from build123d import *

# Parameters (mm, degrees)
SKETCH1_W           = 114.3
SKETCH1_H           = 9.525
BOSS_EXTRUDE1_DEPTH = 3.175
SKETCH2_W           = 9.525
SKETCH2_H           = 63.5
BOSS_EXTRUDE2_DEPTH = 3.175
SKETCH3_W           = 9.525
SKETCH3_H           = 3.81
BOSS_EXTRUDE3_DEPTH = 12.7
SKETCH4_W           = 114.3
SKETCH4_H           = 3.81
BOSS_EXTRUDE4_DEPTH = 3.175
CHAMFER1_SIZE       = 12.7
CHAMFER2_SIZE       = 6.35


with BuildPart() as part:
    # Sketch1 → Boss-Extrude1 (new body)
    with BuildSketch(Plane(origin=(0, 0, 0), x_dir=(1, 0, 0), z_dir=(0, 1, 0))):
        Rectangle(SKETCH1_W, SKETCH1_H)
    extrude(amount=BOSS_EXTRUDE1_DEPTH)

    # Sketch2 → Boss-Extrude2 (add)
    with BuildSketch(Plane(origin=(0, 3.175, 0), x_dir=(1, 0, 0), z_dir=(0, 1, 0))):
        with Locations((-52.3875, 0)):
            Rectangle(SKETCH2_W, SKETCH2_H)
        with Locations((52.3875, 0)):
            Rectangle(SKETCH2_W, SKETCH2_H)
        with Locations((17.4625, 0)):
            Rectangle(SKETCH2_W, SKETCH2_H)
        with Locations((-17.4625, 0)):
            Rectangle(SKETCH2_W, SKETCH2_H)
    extrude(amount=-BOSS_EXTRUDE2_DEPTH)

    # Sketch3 → Boss-Extrude3 (add)
    with BuildSketch(Plane(origin=(0, 3.175, 0), x_dir=(1, 0, 0), z_dir=(0, 1, 0))):
        with Locations((-52.3875, -29.845)):
            Rectangle(SKETCH3_W, SKETCH3_H)
        with Locations((-17.4625, -29.845)):
            Rectangle(SKETCH3_W, SKETCH3_H)
        with Locations((17.4625, -29.845)):
            Rectangle(SKETCH3_W, SKETCH3_H)
        with Locations((52.3875, -29.845)):
            Rectangle(SKETCH3_W, SKETCH3_H)
        with Locations((52.3875, 29.845)):
            Rectangle(SKETCH3_W, SKETCH3_H)
        with Locations((17.4625, 29.845)):
            Rectangle(SKETCH3_W, SKETCH3_H)
        with Locations((-17.4625, 29.845)):
            Rectangle(SKETCH3_W, SKETCH3_H)
        with Locations((-52.3875, 29.845)):
            Rectangle(SKETCH3_W, SKETCH3_H)
    extrude(amount=BOSS_EXTRUDE3_DEPTH)

    # Sketch4 → Boss-Extrude4 (add)
    with BuildSketch(Plane(origin=(0, 15.875, 0), x_dir=(1, 0, 0), z_dir=(0, 1, 0))):
        with Locations((0, -29.845)):
            Rectangle(SKETCH4_W, SKETCH4_H)
        with Locations((0, 29.845)):
            Rectangle(SKETCH4_W, SKETCH4_H)
    extrude(amount=BOSS_EXTRUDE4_DEPTH)

    # Chamfer1
    chamfer1_edges = [part.edges().sort_by_distance(p)[0] for p in [
        (47.625, 15.875, -29.845),
        (22.225, 15.875, -29.845),
        (12.7, 15.875, -29.845),
        (-12.7, 15.875, -29.845),
        (-22.225, 15.875, -29.845),
        (-47.625, 15.875, -29.845),
        (47.625, 15.875, 29.845),
        (22.225, 15.875, 29.845),
        (12.7, 15.875, 29.845),
        (-12.7, 15.875, 29.845),
        (-22.225, 15.875, 29.845),
        (-47.625, 15.875, 29.845),
    ]]
    chamfer(chamfer1_edges, length=CHAMFER1_SIZE - 0.0001)  # a hair under: the kernel refuses the full size

    # Chamfer2
    chamfer2_edges = [part.edges().sort_by_distance(p)[0] for p in [
        (-52.3875, 3.175, -27.94),
        (-17.4625, 3.175, -27.94),
        (17.4625, 3.175, -27.94),
        (52.3875, 3.175, -27.94),
        (52.3875, 3.175, 27.94),
        (17.4625, 3.175, 27.94),
        (-17.4625, 3.175, 27.94),
        (-52.3875, 3.175, 27.94),
    ]]
    chamfer(chamfer2_edges, length=CHAMFER2_SIZE)
    chamfer2_2_edges = [part.edges().sort_by_distance(p)[0] for p in [
        (-52.3875, 0, -31.75),
        (-17.4625, 0, -31.75),
        (17.4625, 0, -31.75),
        (52.3875, 0, -31.75),
        (52.3875, 0, 31.75),
        (17.4625, 0, 31.75),
        (-17.4625, 0, 31.75),
        (-52.3875, 0, 31.75),
    ]]
    chamfer(chamfer2_2_edges, length=CHAMFER2_SIZE)


solid = part.part
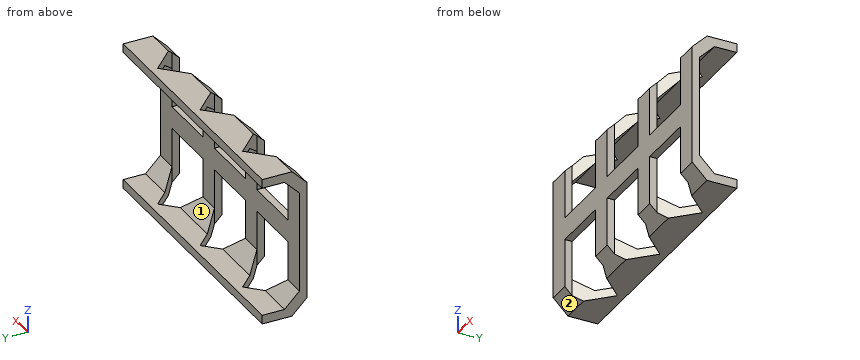
Here's how the part is built. I have some questions about the finished solid (model axes, mm). Face numbers are marked on the shaded views. A direction names the side the tool comes from. Round coordinates to 2 decimals unless told otherwise and drop trailing zeros. Write each loop counter-clockwise with the first axis right and the second up, starting at its lowest first coordinate (ties: lowest second). Pieces come first, ordered by that corner, then holes.
1. I need wall thicknesses on L1, parallel to X at y = 1.25, z = -21.5 (3 decimals); L2, parallel to Z at x = -48.5, y = 16.5; L3, parallel to Z at x = 44.5, y = 7 (3 decimals). Which ranges of each line are inside material? Lowest first, please.
2. For the marked faces 1 and 2, which set-ups out of +Z, -Z, +X, -X, +Y, -Y let a thin tool reach every point of the face, with its end or its side?
3. Suppose I cut it at A-A (z = 13.5). List the corners of the cut face in (x, y) for me (3 decimals), and give its area (3 significant figures).
4. Will these pins go through, and if not, where does the flat tip stop? pin 1 Ø10 at (y, z) = (8.5, -9.5) entering from +X; pin 2 Ø3 at (x, y) = (-7.5, 8) entering from -Z; pin 3 Ø3.5 at (x, y) = (33, 1) entering from +Z; pin 4 Ø2.5 at (x, y) = (-5, 1) entering from -Z.
5. Suppose I cut it at B-B (y = 4.5). State how many separate pieces and enclosed holes the cut face has, and give its area (3 significant figures).
Answer sheet:
1. L1: x = -57.15 to -47.625, -22.225 to -12.7, 12.7 to 22.225, 47.625 to 57.15
1. L2: z = -31.75 to -27.94, 27.94 to 31.75
1. L3: z = -31.75 to -25.415, 25.415 to 31.75
2. face 1: +X, -X, +Y
2. face 2: -Z, +X, -X, -Y
3. outline: (-57.15, 0) - (-47.625, 0) - (-47.625, 3.175) - (-57.15, 3.175) - close; (-22.225, 0) - (-12.7, 0) - (-12.7, 3.175) - (-22.225, 3.175) - close; (12.7, 0) - (22.225, 0) - (22.225, 3.175) - (12.7, 3.175) - close; (47.625, 0) - (57.15, 0) - (57.15, 3.175) - (47.625, 3.175) - close
3. area: 121 mm2
4. pin 1: passes through
4. pin 2: stops at z = -31.75
4. pin 3: stops at z = 4.76
4. pin 4: stops at z = -4.76
5. separate pieces: 8
5. enclosed holes: 0
5. area: 643 mm2
